Geometry: final body of the model. Coordinates: model frame, mm. A direction names the side the tool comes from. Coordinates: 2 decimals unless noted, no trailing zeros. Order: outer loops, then holes, each group sorted by start corner. A loop starts at its lowest first (then second) coordinate and runs counter-clockwise, first axis right, second up. Notation, with made-up numbers: (-9, 59.5) - (-2, 59.5) arc R25 cw to (-2, 86.5) - close; hole circle Ø9 at (80, -3). An arc over 180 degrees is marked (long way). Use a Markdown table: item, result. Add a question column.
Autodesk Inventor part; units mm, degrees
ref_plane "YZ Plane" through (0, 0, 0) normal (1, 0, 0) x (0, 1, 0)
ref_plane "XZ Plane" through (0, 0, 0) normal (0, 1, 0) x (-1, 0, 0)
ref_plane "XY Plane" through (0, 0, 0) normal (0, 0, 1) x (1, 0, 0)
sketch "Sketch1" plane through (0, 0, 0) normal (0, 1, 0) x (-1, 0, 0)
  line L0 (58.8, 0) -> (0, 0)
  line L1 (0, 0) -> (0, -32)
  line L2 (0, -32) -> (58.8, -32)
  line L3 (58.8, -32) -> (58.8, 0)
  line L4 (41.9, -3.5) -> (16.9, -3.5) construction
  line L5 (16.9, -3.5) -> (16.9, -28.5) construction
  line L6 (16.9, -28.5) -> (41.9, -28.5) construction
  line L7 (41.9, -28.5) -> (41.9, -3.5) construction
  circle A0 centre (41.9, -3.5) radius 1.5
  circle A1 centre (16.9, -3.5) radius 1.5
  circle A2 centre (41.9, -28.5) radius 1.5
  circle A3 centre (16.9, -28.5) radius 1.5
  point P0 (41.9, -16)
  point P1 (58.8, -16)
  point P2 (29.4, -28.5)
  point P3 (29.4, -32)
  dimension "d0" = 3
  dimension "d1" = 25
  dimension "d2" = 32
  dimension "d3" = 58.8
extrude "Extrusion1" add sketch "Sketch1" along normal blind 2
sketch "Sketch2" plane through (-58.8, 0, -32) normal (-1, 0, 0) x (0, 0, 1)
  circle A0 centre (31, 17.2) radius 16 construction
  circle A1 centre (42.3137, 28.5137) radius 2.4
  circle A2 centre (15, 17.2) radius 2.4
  circle A3 centre (19.6863, 5.8863) radius 2.4
  circle A4 centre (19.6863, 28.5137) radius 2.4
  circle A5 centre (47, 17.2) radius 2.4
  circle A6 centre (42.3137, 5.8863) radius 2.4
  line L0 (19.6863, 28.5137) -> (42.3137, 5.8863) construction
  line L1 (15, 17.2) -> (31, 17.2) construction
  line L2 (0, 2) -> (32, 2)
  arc A7 (43.0482, 0) -> (16.51, 2) centre (31, 17.2) ccw
  line L3 (0, 0) -> (32, 0)
  line L4 (32, 0) -> (43.0482, 0)
  line L5 (32, 0) -> (32, 2)
  line L6 (0, 2) -> (0, 38.2)
  line L7 (0, 38.2) -> (31, 38.2)
  circle A8 centre (31, 17.2) radius 6.25
  line L8 (31, 38.2) -> (62, 38.2)
  line L9 (62, 38.2) -> (62, 0)
  line L10 (32, 0) -> (0, 0)
  line L11 (62, 0) -> (32, 0)
  point P0 (31, 17.2)
  dimension "d6" = 4.8
  dimension "d7" = 32
  dimension "d9" = 15.2
  dimension "d11" = 45
  dimension "d12" = 31
  dimension "d14" = 21
  dimension "d17" = 12.5
  dimension "d29" = 31
extrude "Extrusion2" add sketch "Sketch2" against normal up to surface (58.8 mm away) contours L6 L7 A7 L2 | A7 L4 L5 L2
sketch "Sketch3" plane through (-58.8, 0, -32) normal (-1, 0, 0) x (0, 0, 1)
  circle A0 centre (31, 17.2) radius 10.025
  circle A1 centre (31, 17.2) radius 6.25 construction
  point P0 (32, 0)
  dimension "d18" = 20.05
extrude "Extrusion3" cut sketch "Sketch3" against normal blind 27.05
sketch "Sketch4" plane through (-58.8, 38.2, -1) normal (0, 1, 0) x (1, 0, 0)
  circle A0 centre (41.9, 2.5) radius 1.5
  circle A1 centre (41.9, 27.5) radius 1.5
  circle A2 centre (16.9, 2.5) radius 1.5
  circle A3 centre (16.9, 27.5) radius 1.5
  circle A4 centre (16.9, 2.5) radius 3
  circle A5 centre (16.9, 27.5) radius 3
  circle A6 centre (41.9, 27.5) radius 3
  circle A7 centre (41.9, 2.5) radius 3
  point P0 (58.8, -1)
  dimension "d21" = 6
extrude "Extrusion4" cut sketch "Sketch4" against normal up to surface (36.2 mm away) contours A0 | A1 | A2 | A3 | A4 | A5 | A6 | A7
sketch "Sketch5" plane through (0, 0, -32) normal (0, 0, -1) x (-1, 0, 0)
  circle A0 centre (49.4, 6.6) radius 2.85
  circle A1 centre (9.4, 6.6) radius 2.85
  circle A2 centre (49.4, 31.6) radius 2.85
  circle A3 centre (9.4, 31.6) radius 2.85
  line L0 (49.4, 31.6) -> (9.4, 31.6) construction
  line L1 (9.4, 31.6) -> (9.4, 6.6) construction
  line L2 (9.4, 6.6) -> (49.4, 6.6) construction
  line L3 (49.4, 6.6) -> (49.4, 31.6) construction
  line L4 (58.8, 38.2) -> (0, 38.2) construction
  line L5 (0, 0) -> (0, 38.2) construction
  point P0 (29.4, 31.6)
  point P1 (29.4, 38.2)
  point P2 (9.4, 19.1)
  point P3 (0, 19.1)
  dimension "d24" = 5.7
  dimension "d25" = 40
  dimension "d26" = 25
extrude "Extrusion5" cut sketch "Sketch5" against normal blind 15
sketch "Sketch6" plane through (-58.8, 0, -32) normal (-1, 0, 0) x (0, 0, 1)
  arc A0 (43.0482, 0) -> (31, 38.2) centre (31, 17.2) ccw
  line L0 (31, 38.2) -> (62, 38.2)
  line L1 (62, 38.2) -> (62, 0)
  line L2 (43.0482, 0) -> (0, 0)
  line L3 (62, 0) -> (43.0482, 0)
  point P0 (32, 0)
  dimension "d30" = 31
extrude "Extrusion6" add sketch "Sketch6" against normal up to surface (58.8 mm away)
ref_plane "Work Plane1" through (0, 38.2, -1) normal (0, 0, -1) x (-1, 0, 0)
mirror "Mirror1" about plane through (0, 38.2, -1) normal (0, 0, -1) of "Extrusion5"
properties part number "X_Axis_Connector"
1) Section A-A (y = 17.2). Return loops of the section in (x, z) (3 decimals).
2) Pin query (flat end, axial travel): pin 1 (3 mm diameter, centred on x = -9.5, y = 31.5, fed in from +Z); pin 2 (2.5 mm diameter, centred on x = -16.9, z = -3.5, fed in from -Y); pin 3 (3.5 mm diameter, centred on x = -49.4, y = 31.6, fed in from -Z); pin 4 (7 mm diameter, centred on x = -16.9, z = -3.5, fed in from -Y). Return the tip coordinate at first contact, or that it passes through.
3) Section C-C (z = -13). Return loops of the section in (x, y), then the cut area to 3 significant figures.
4) Set-up query: faces 1 (the face through (-31.75, 13, -6)), 2 (the face through (-39.04, 20.35, -29.4)), 3 (the face through (-10.932, 29.197, 22.605)), 4 (the face through (-9, 32, -17)). Return all of +Z, -Z, +X, -X, +Y, -Y with unobstructed straight access to the full face (end or side cutting, diameter ignored); none if empty.
5) Draft query along Y for faces 5 (the face through (-30, 38.2, -1)), 6 (the face through (-17.291, 6.843, -6.474)), 7 (the face through (-30, 19, 30)). Return one class per face: pulls with the +Y half, pulls with the -Y half, needs draft (parallel to the pull), parting line crosses it, or undercut.
6) Ray query, line 1 along Z through (x, y) = (-3.5, 6); line 2 along Z through (x, y) = (-41.9, 17.5); line 3 along X through (y, z) = (19, -28.5). Return the intervals inside material, ascending.
7) Section B-B (x = -41.9). Give the number of separate pieces and of enclosed holes in the cut face, then the cut area to 3 significant figures.
Values follow:
| question | item | result |
|---|---|---|
| 1 | outline | (-58.8, -32) - (0, -32) - (0, -19.4) - (-58.8, -19.4) - close; (-58.8, -14.6) - (0, -14.6) - (0, -7.25) - (-31.75, -7.25) - (-31.75, -11.025) - (-58.8, -11.025) - close; (-58.8, 9.025) - (-31.75, 9.025) - (-31.75, 5.25) - (0, 5.25) - (0, 12.6) - (-58.8, 12.6) - close; (-58.8, 17.4) - (0, 17.4) - (0, 30) - (-58.8, 30) - close; hole circle Ø6 at (-41.9, -28.5); hole circle Ø6 at (-16.9, -28.5) |
| 2 | pin 1 | stops at z = 15 |
| 2 | pin 2 | passes through |
| 2 | pin 3 | stops at z = -17 |
| 2 | pin 4 | stops at y = 0 |
| 3 | outline | (-58.8, 0) - (0, 0) - (0, 3.59) - (-58.8, 3.59) - close; (-58.8, 8.19) - (0, 8.19) - (0, 26.21) - (-58.8, 26.21) - close; (-58.8, 30.81) - (0, 30.81) - (0, 38.2) - (-58.8, 38.2) - close |
| 3 | area | 1,710 mm² |
| 4 | face 1 | -X |
| 4 | face 2 | +Y |
| 4 | face 3 | +Z |
| 4 | face 4 | -Z |
| 5 | face 5 | pulls with the +Y half |
| 5 | face 6 | undercut |
| 5 | face 7 | needs draft |
| 6 | line 1 | z = -32 to -14.71, -9.92 to 7.92, 12.71 to 30 |
| 6 | line 2 | z = -32 to -31.5, -25.5 to -19.38, -14.62 to -11.02, 9.02 to 12.62, 17.38 to 30 |
| 6 | line 3 | x = -58.8 to -44.9, -38.9 to -19.9, -13.9 to 0 |
| 7 | separate pieces | 3 |
| 7 | enclosed holes | 6 |
| 7 | area | 1,610 mm² |
